Here's the drawing with two shaded views (mm, measured from the low corner). I have some questions. A direction names the side the tool comes from. Give positions to 0.01 mm unless a question says otherwise; leave off trailing zeros. Loops run counter-clockwise (first coordinate to the right, second up) from the corner with the lowest first, then second, coordinate; pieces in that order, holes last. Notation, with made-up numbers: (-5, -1) -> (39, -1) arc R35 cw to (39, 34) -> close; hole circle Ø4 at (52.5, -15.75). An arc over 180 degrees is marked (long way). Write each question's results on one line, items separated by ' | '. Start each with the question number.
Q1. Which directions (+Z, -Z, +X, -X, +Y, -Y) give clear straight access to the entire face, cutting with the end or side of a thin tool? Please do the marked faces 1 and 2.
Q2. If we section it at C-C, the plane z = 61: List the corners of the cut face in (x, y) for me.
Q3. If we section it at A-A, the plane x = 34: List the corners of the cut face in (y, z) for me, plus the area to 3 significant figures.
Q4. If I drill on line 1 along Y through (x, z) = (8.5, 28); line 2 along Z through (x, y) = (7, 6); line 3 along Z through (x, y) = (34, 58.5), over which ranges is the centre line in solid material (lowest first)?
Q5. If we section it at B-B, the plane z = 34: List the corners of the cut face in (x, y) for me.
Q6. Will these pins go through, and if not, where does the flat tip stop? P1, Ø8, axis at x = 7, z = 34, coming from the +Y side; P2, Ø4, axis at x = 14.5, z = 18, coming from the -Y side; P3, Ø1.5, axis at x = 29, y = 87.5, coming from the -Z side; P4, Ø12, axis at y = 105.5, z = 32, coming from the -X side.
Q7. If we section it at D-D, the plane x = 61: List the corners of the cut face in (y, z) for me, plus the area to 3 significant figures.
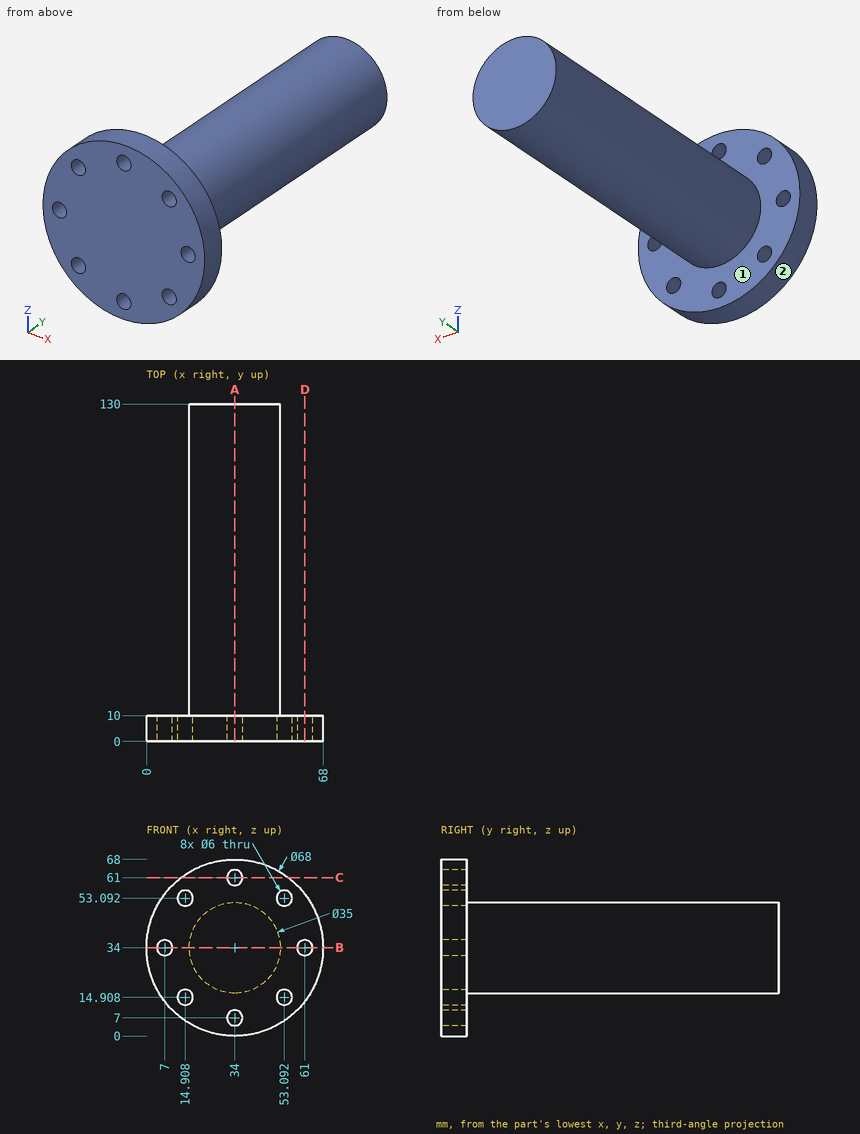
Final values:
1) face 1: +Y | face 2: +Y, -Y
2) outline: (13.34, 0) -> (31, 0) -> (31, 10) -> (13.34, 10) -> close; (37, 0) -> (54.66, 0) -> (54.66, 10) -> (37, 10) -> close
3) outline: (0, 0) -> (10, 0) -> (10, 4) -> (0, 4) -> close; (0, 10) -> (10, 10) -> (10, 16.5) -> (130, 16.5) -> (130, 51.5) -> (10, 51.5) -> (10, 58) -> (0, 58) -> close; (0, 64) -> (10, 64) -> (10, 68) -> (0, 68) -> close | area: 4,760 mm²
4) line 1: y = 0 to 10 | line 2: z = 13.34 to 31, 37 to 54.66 | line 3: z = 16.5 to 51.5
5) outline: (0, 0) -> (4, 0) -> (4, 10) -> (0, 10) -> close; (10, 0) -> (58, 0) -> (58, 10) -> (51.5, 10) -> (51.5, 130) -> (16.5, 130) -> (16.5, 10) -> (10, 10) -> close; (64, 0) -> (68, 0) -> (68, 10) -> (64, 10) -> close
6) P1: stops at y = 10 | P2: stops at y = 0 | P3: stops at z = 17.02 | P4: stops at x = 16.5
7) outline: (0, 13.34) -> (10, 13.34) -> (10, 31) -> (0, 31) -> close; (0, 37) -> (10, 37) -> (10, 54.66) -> (0, 54.66) -> close | area: 353 mm²
